```python
from build123d import *

# Parameters (mm, degrees)
SKETCH_1_R               = 156
EXTRUDE_1_DEPTH          = 10
SKETCH_2_R               = 2.6
CUT_EXTRUDE_1_DEPTH      = 221.843836228
SKETCH_3_R               = 40.05
CUT_EXTRUDE_2_DEPTH      = 10
SKETCH_4_R               = 2.6
CUT_EXTRUDE_4_DEPTH      = 221.843836228
PATTERN_CIRCULAR_1_COUNT = 6


with BuildPart() as part:
    # Эскиз1 → Бобышка-Вытянуть1 (new body)
    with BuildSketch(Plane(origin=(0, 0, 0), x_dir=(1, 0, 0), z_dir=(0, 1, 0))):
        with Locations(Location((0, 0, 0), (0, 0, 270))):
            Circle(SKETCH_1_R)
    extrude(amount=EXTRUDE_1_DEPTH)

    # Эскиз2 → Вырез-Вытянуть1 (cut, through all)
    with BuildSketch(Plane(origin=(0, 10, 0), x_dir=(1, 0, 0), z_dir=(0, 1, 0))):
        with Locations(Location((116, 13.8, 0), (0, 0, 270))):
            Circle(SKETCH_2_R)
        with Locations(Location((116, 53.8, 0), (0, 0, 270))):
            Circle(SKETCH_2_R)
        with Locations(Location((116, -26.2, 0), (0, 0, 270))):
            Circle(SKETCH_2_R)
        with Locations(Location((116, -66.2, 0), (0, 0, 270))):
            Circle(SKETCH_2_R)
        with Locations(Location((-116, -66.2, 0), (0, 0, 90))):
            Circle(SKETCH_2_R)
        with Locations(Location((-116, -26.2, 0), (0, 0, 90))):
            Circle(SKETCH_2_R)
        with Locations(Location((-116, 13.8, 0), (0, 0, 90))):
            Circle(SKETCH_2_R)
        with Locations(Location((-116, 53.8, 0), (0, 0, 90))):
            Circle(SKETCH_2_R)
    extrude(amount=-CUT_EXTRUDE_1_DEPTH, mode=Mode.SUBTRACT)

    # Эскиз3 → Вырез-Вытянуть2 (cut)
    with BuildSketch(Plane(origin=(0, 10, 0), x_dir=(1, 0, 0), z_dir=(0, 1, 0))):
        with Locations(Location((0, 0, 0), (0, 0, 270))):
            Circle(SKETCH_3_R)
    extrude(amount=-CUT_EXTRUDE_2_DEPTH, mode=Mode.SUBTRACT)

    # Эскиз4 → Вырез-Вытянуть4 (cut, through all)
    with BuildSketch(Plane(origin=(0, 10, 0), x_dir=(1, 0, 0), z_dir=(0, 1, 0))):
        with Locations(Location((-135, 0, 0), (0, 0, 270))):
            Circle(SKETCH_4_R)
    cut_extrude_4 = extrude(amount=-CUT_EXTRUDE_4_DEPTH, mode=Mode.SUBTRACT)

    # Круговой массив1: Вырез-Вытянуть4 ×6 about axis
    pattern_circular_1_axis = Axis((0, 0, 0), (0, 1, 0))
    for i in range(1, PATTERN_CIRCULAR_1_COUNT):
        add(cut_extrude_4.rotate(pattern_circular_1_axis, i * 360 / PATTERN_CIRCULAR_1_COUNT), mode=Mode.SUBTRACT)


solid = part.part
```
Here's how the part is built. I have some questions about the finished solid (model axes, mm). Coordinates: 2 decimals unless noted, no trailing zeros. Write each loop counter-clockwise with the first axis right and the second up, starting at its lowest first coordinate (ties: lowest second). Pieces come first, ordered by that corner, then holes. Notation, with made-up numbers: (22.5, 65) -> (36.5, 65) arc R20 cw to (36.5, 72) -> close; hole circle Ø10 at (-13, -38). An arc over 180 degrees is marked (long way). Use a Markdown table: item, result. Add a question column.
(1) If we section it at B-B, the plane z = 15: Write out the boundary of the cut face in (x, y), and give its area (3 significant figures).
(2) If we section it at C-C, the plane y = 2: State how many separate pieces and enclosed holes the cut face has, and give its area (3 significant figures).
(3) We'd pull the mould along Z, two halves only. Please class faces 1 (the cylindrical face through (-39.1, 5.07, -8.68)), 2 (the cylindrical face through (154.672, 4.93, -20.308)), 3 (the flat face through (-32, 0, 32)): +Z half, -Z half, draft (parallel to the pull), parting line (faces both ways), or undercut.
(4) I'm going to push flat-ended pins straight in: P1, Ø5, axis at y = 4, z = 39, coming from the -X side; P2, Ø3, axis at x = 5, z = 77.5, coming from the -Y side; P3, Ø4, axis at y = 7.5, z = 79, coming from the +X side; P4, Ø5, axis at y = 5, z = 112, coming from the +X side. Where does each tip first touch, or does it pass through?
(5) If we section it at A-A, the plane x = 0: Write out the boundary of the cut face in (y, z), and give its area (3 significant figures).
(6) If we section it at D-D, the plane x = -53.5: Write out the boundary of the cut face in (y, z), and give its area (3 significant figures).
(7) Please list where these lines run through material, in increasing order: line 1 (X direction, y = 3.25, z = 0); line 2 (X direction, y = 1, z = 118); line 3 (X direction, y = 6.5, z = 66.2).
Outcome:
| question | item | result |
|---|---|---|
| 1 | outline | (-155.28, 0) -> (-37.13, 0) -> (-37.13, 10) -> (-155.28, 10) -> close; (37.13, 0) -> (155.28, 0) -> (155.28, 10) -> (37.13, 10) -> close |
| 1 | area | 2,360 mm^2 |
| 2 | separate pieces | 1 |
| 2 | enclosed holes | 15 |
| 2 | area | 71,100 mm^2 |
| 3 | face 1 | undercut |
| 3 | face 2 | parting line |
| 3 | face 3 | draft |
| 4 | P1 | stops at x = -151.67 |
| 4 | P2 | stops at y = 0 |
| 4 | P3 | stops at x = 135.67 |
| 4 | P4 | stops at x = 111.11 |
| 5 | outline | (0, -156) -> (10, -156) -> (10, -40.05) -> (0, -40.05) -> close; (0, 40.05) -> (10, 40.05) -> (10, 156) -> (0, 156) -> close |
| 5 | area | 2,320 mm^2 |
| 6 | outline | (0, -146.54) -> (10, -146.54) -> (10, 146.54) -> (0, 146.54) -> close |
| 6 | area | 2,930 mm^2 |
| 7 | line 1 | x = -156 to -137.6, -132.4 to -40.05, 40.05 to 132.4, 137.6 to 156 |
| 7 | line 2 | x = -102.04 to -69.86, -65.14 to 65.14, 69.86 to 102.04 |
| 7 | line 3 | x = -141.26 to -118.6, -113.4 to 113.4, 118.6 to 141.26 |
